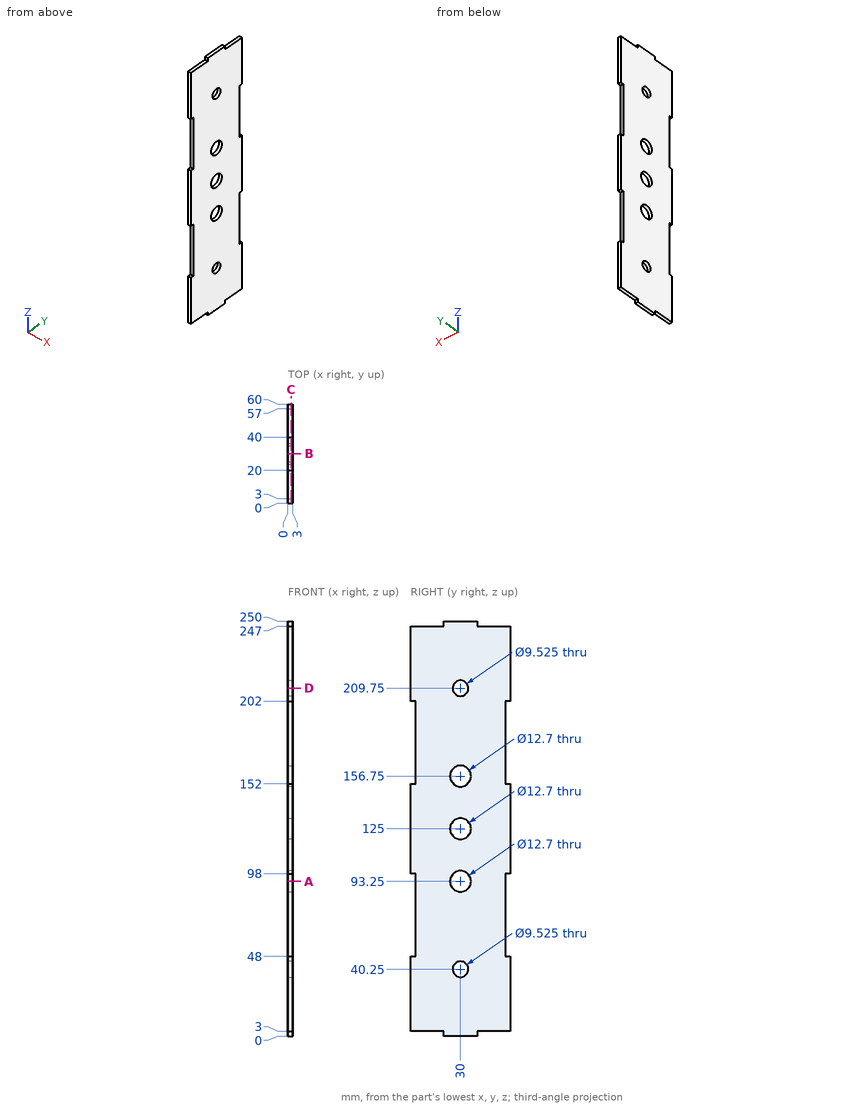
Print and shaded views of the part. All mm, measured from the part's lowest x, y and z. Coordinates: 2 decimals unless noted, no trailing zeros. Order: outer loops, then holes, each group sorted by start corner. A loop starts at its lowest first (then second) coordinate and runs counter-clockwise, first axis right, second up. Notation, with made-up numbers: M 9.5,83 L 59.5,83 A24 cw 59.5,94 Z; hole C 48.25,-3 d11. An arc over 180 degrees is marked long. One line per question, with ' | ' between items. Start each with the question number.
Q1. Saw through at A-A (z = 93.25). List the corners of the cut face in (x, y).
Q2. Saw through at C-C (x = 2). Count the separate pieces of the cut face and the enclosed holes in it, then the cut area to 3 significant figures.
Q3. Flat gauge pins, fed straight in: pin 1 Ø1.5 at (x, y) = (1.5, 1) entering from -Z; pin 2 Ø10 at (y, z) = (30, 93.25) entering from +X; pin 3 Ø0.9 at (x, z) = (1, 2) entering from +Y; pin 4 Ø0.9 at (x, z) = (1.5, 177.5) entering from +Y. Where does each tip first touch, or does it go through?
Q4. Saw through at B-B (y = 30). List the corners of the cut face in (x, z).
Q5. Probe L1, parallel to Y at x = 1.8, z = 93.25; L2, parallel to Y at x = 2.2, z = 40.25; L3, parallel to Y at x = 2.7, z = 72.5. List the from-to ranges inside material, lowest first. Write a range as from..to.
Q6. Saw through at D-D (z = 209.75). List the corners of the cut face in (x, y), then the cut area to 3 significant figures.
Check values:
1) outline: M 0,3 L 3,3 L 3,23.65 L 0,23.65 Z; M 0,36.35 L 3,36.35 L 3,57 L 0,57 Z
2) separate pieces: 1 | enclosed holes: 5 | area: 13,600 mm2
3) pin 1: stops at z = 3 | pin 2: passes through | pin 3: stops at y = 40 | pin 4: stops at y = 57
4) outline: M 0,0 L 3,0 L 3,35.49 L 0,35.49 Z; M 0,45.01 L 3,45.01 L 3,86.9 L 0,86.9 Z; M 0,99.6 L 3,99.6 L 3,118.65 L 0,118.65 Z; M 0,131.35 L 3,131.35 L 3,150.4 L 0,150.4 Z; M 0,163.1 L 3,163.1 L 3,204.99 L 0,204.99 Z; M 0,214.51 L 3,214.51 L 3,250 L 0,250 Z
5) L1: y = 3..23.65, 36.35..57 | L2: y = 0..25.24, 34.76..60 | L3: y = 3..57
6) outline: M 0,0 L 3,0 L 3,25.24 L 0,25.24 Z; M 0,34.76 L 3,34.76 L 3,60 L 0,60 Z | area: 151 mm2
